Autodesk Inventor part; units mm, degrees
ref_plane "YZ Plane" through (0, 0, 0) normal (1, 0, 0) x (0, 1, 0)
ref_plane "XZ Plane" through (0, 0, 0) normal (0, 1, 0) x (-1, 0, 0)
ref_plane "XY Plane" through (0, 0, 0) normal (0, 0, 1) x (1, 0, 0)
sketch "Sketch1" plane through (0, 0, 0) normal (0, 1, 0) x (-1, 0, 0)
  line L0 (4.0726, -0.3796) -> (56.5523, -0.3796) construction
  line L1 (56.5523, -0.3796) -> (56.5523, -20.3796) construction
  line L2 (56.5523, -20.3796) -> (4.0726, -20.3796) construction
  line L3 (4.0726, -20.3796) -> (4.0726, -0.3796) construction
  line L4 (20.1018, -0.3796) -> (13.3433, -11.5303)
  line L5 (13.3433, -11.5303) -> (13.3433, -20.3796)
  line L6 (13.3433, -20.3796) -> (10.6852, -20.3796)
  line L7 (10.6852, -20.3796) -> (10.6852, -11.8059)
  line L8 (10.6852, -11.8059) -> (3.9267, -0.3796)
  line L9 (3.9267, -0.3796) -> (6.8765, -0.3796)
  line L10 (6.8765, -0.3796) -> (12.0305, -9.1803)
  line L11 (12.0305, -9.1803) -> (17.2817, -0.3796)
  line L12 (17.2817, -0.3796) -> (20.1018, -0.3796)
  line L13 (39.0969, -20.3796) -> (36.4389, -20.3796)
  line L14 (36.4389, -20.3796) -> (36.4389, -3.1511)
  line L15 (36.4389, -3.1511) -> (31.2201, -14.8691)
  line L16 (31.2201, -14.8691) -> (29.5993, -14.8691)
  line L17 (29.5993, -14.8691) -> (24.4292, -3.1511)
  line L18 (24.4292, -3.1511) -> (24.4292, -20.3796)
  line L19 (24.4292, -20.3796) -> (21.9494, -20.3796)
  line L20 (21.9494, -20.3796) -> (21.9494, -0.3796)
  line L21 (21.9494, -0.3796) -> (25.5799, -0.3796)
  line L22 (25.5799, -0.3796) -> (30.5718, -11.5141)
  line L23 (30.5718, -11.5141) -> (35.4016, -0.3796)
  line L24 (35.4016, -0.3796) -> (39.0969, -0.3796)
  line L25 (39.0969, -0.3796) -> (39.0969, -20.3796)
  line L26 (43.1488, -20.3796) -> (43.1488, -0.3796)
  line L27 (43.1488, -0.3796) -> (55.6609, -0.3796)
  line L28 (55.6609, -0.3796) -> (55.6609, -2.7459)
  line L29 (55.6609, -2.7459) -> (45.8068, -2.7459)
  line L30 (45.8068, -2.7459) -> (45.8068, -8.224)
  line L31 (45.8068, -8.224) -> (54.9964, -8.224)
  line L32 (54.9964, -8.224) -> (54.9964, -10.5903)
  line L33 (54.9964, -10.5903) -> (45.8068, -10.5903)
  line L34 (45.8068, -10.5903) -> (45.8068, -18.0133)
  line L35 (45.8068, -18.0133) -> (55.6609, -18.0133)
  line L36 (55.6609, -18.0133) -> (55.6609, -20.3796)
  line L37 (55.6609, -20.3796) -> (43.1488, -20.3796)
  point P0 (0, 0)
extrude "Extrusion1" add sketch "Sketch1" along normal blind 5
sketch "Sketch2" plane through (0, 5, 0) normal (0, 1, 0) x (1, 0, 0)
  line L0 (-17.2817, 0.3796) -> (-12.0305, 9.1803)
  line L1 (-55.6609, 0.3796) -> (-43.1488, 0.3796)
  line L2 (-17.2817, 0.3796) -> (-20.1018, 0.3796)
  line L3 (-55.6609, 2.7459) -> (-55.6609, 0.3796)
  line L4 (-55.6609, 0.3796) -> (-55.6609, 2.7459)
  line L5 (-55.6609, 2.7459) -> (-16.2934, 2.7459)
  line L6 (-16.2934, 2.7459) -> (-17.3426, 0.3796)
  line L7 (-13.3433, 11.5303) -> (-20.1018, 0.3796)
  line L8 (-20.1018, 0.3796) -> (-24.9933, 0.3796)
  line L9 (-21.9494, 0.3796) -> (-25.5799, 0.3796)
  line L10 (-26.1142, 2.7459) -> (-24.9933, 0.3796)
  line L11 (-55.6609, 0.3796) -> (-38.2567, 0.3796)
  line L12 (-39.0969, 0.3796) -> (-35.4016, 0.3796)
  line L13 (-38.2567, 2.7459) -> (-49.9322, 2.7459)
  line L14 (-38.2567, 0.3796) -> (-38.2567, 2.7459)
  point P0 (0, 0)
extrude "Extrusion2" add sketch "Sketch2" against normal blind 5
sketch "Sketch3" plane through (0, 5, 0) normal (0, 1, 0) x (1, 0, 0)
  line L0 (-6.8765, 0.3796) -> (-3.9267, 0.3796)
  line L1 (-6.8765, 0.3796) -> (-1.8765, 0.3796)
  line L2 (-1.8765, 0.3796) -> (-1.8765, 5.3796)
  line L3 (-1.8765, 5.3796) -> (-6.8765, 5.3796)
  line L4 (-6.8765, 5.3796) -> (-6.8765, 0.3796)
  point P0 (0, 0)
  dimension "d9" = 5
  dimension "d10" = 5
extrude "Extrusion3" add sketch "Sketch3" against normal blind 5
sketch "Sketch4" plane through (0, 5, 0) normal (0, 1, 0) x (1, 0, 0)
  circle A0 centre (-4.3765, 2.8796) radius 1.5
  line L0 (-6.8765, 0.3796) -> (-1.8765, 0.3796)
  line L1 (-1.8765, 0.3796) -> (-1.8765, 5.3796)
  point P0 (0, 0)
  dimension "d6" = 2.5
  dimension "d11" = 2.5
  dimension "d12" = 3
extrude "Extrusion4" cut sketch "Sketch4" against normal blind 5
properties part number "YME"
The listing builds one solid part. Answer for the finished solid, in the listing's coordinates (mm). A direction names the side the tool comes from. Give positions to 0.01 mm unless a question says otherwise; leave off trailing zeros. Write each loop counter-clockwise with the first axis right and the second up, starting at its lowest first coordinate (ties: lowest second). Pieces come first, ordered by that corner, then holes. Notation, with made-up numbers: (-1, 85.25) -> (34, 85.25) arc R22 cw to (34, 122.25) -> close; hole circle Ø6 at (14.25, 47). An arc over 180 degrees is marked (long way). Write item = value, one per line. Start each with the question number.
1) The part is cut by section B-B, the plane z = -15.75. Determine the outline of the cut face in (x, y).
2) The part is cut by section D-D, the plane x = -20.5. Determine the outline of the cut face in (y, z), and give its area (3 significant figures).
3) The part is cut by section A-A, the plane x = -52. Determine the outline of the cut face in (y, z).
4) The part is cut by section C-C, the plane z = -13.25. Determine the outline of the cut face in (x, y), and give its area (3 significant figures).
5) Straight lines are drawn through the part: line 1 along Z through (x, y) = (-50, 3.6); line 2 along X through (y, z) = (2.85, -18.75); line 3 along X through (y, z) = (1.7, -17). For each, find the intervals that lie inside material, in ascending order.
6) Each of these flat-tipped pins is pushed along its axis until it touches: pin 1 (2.5 mm diameter, centred on y = 3, z = -9, fed in from -X); pin 2 (1.5 mm diameter, centred on y = 3, z = -14.5, fed in from -X); pin 3 (3 mm diameter, centred on x = -12.5, y = 3.5, fed in from +Z). Where does it stop, or does it pass through?
7) Which of the six approach directions +Z, -Z, +X, -X, +Y, -Y give full straight-line access (tool end or side, diameter ignored) to faces 1 (the face through (-16.04, 2.46, -7.08)), 2 (the face through (-14.62, 2.46, -4.84)), 3 (the face through (-50, 2, -10.59)), 4 (the face through (-12, 2, -20.38))?
Solutions:
q1.outline = (-45.81, 0) -> (-43.15, 0) -> (-43.15, 5) -> (-45.81, 5) -> close; (-39.1, 0) -> (-36.44, 0) -> (-36.44, 5) -> (-39.1, 5) -> close; (-24.43, 0) -> (-21.95, 0) -> (-21.95, 5) -> (-24.43, 5) -> close; (-13.34, 0) -> (-10.69, 0) -> (-10.69, 5) -> (-13.34, 5) -> close
q2.outline = (0, -2.75) -> (5, -2.75) -> (5, -0.38) -> (0, -0.38) -> close
q2.area = 11.8 mm²
q3.outline = (0, -20.38) -> (5, -20.38) -> (5, -18.01) -> (0, -18.01) -> close; (0, -10.59) -> (5, -10.59) -> (5, -8.22) -> (0, -8.22) -> close; (0, -2.75) -> (5, -2.75) -> (5, -0.38) -> (0, -0.38) -> close
q4.outline = (-45.81, 0) -> (-43.15, 0) -> (-43.15, 5) -> (-45.81, 5) -> close; (-39.1, 0) -> (-36.44, 0) -> (-36.44, 5) -> (-39.1, 5) -> close; (-31.94, 0) -> (-28.88, 0) -> (-28.88, 5) -> (-31.94, 5) -> close; (-24.43, 0) -> (-21.95, 0) -> (-21.95, 5) -> (-24.43, 5) -> close; (-13.34, 0) -> (-10.69, 0) -> (-10.69, 5) -> (-13.34, 5) -> close
q4.area = 67.6 mm²
q5.line_1 = -20.38 to -18.01, -10.59 to -8.22, -2.75 to -0.38
q5.line_2 = -55.66 to -43.15, -39.1 to -36.44, -24.43 to -21.95, -13.34 to -10.69
q5.line_3 = -45.81 to -43.15, -39.1 to -36.44, -24.43 to -21.95, -13.34 to -10.69
q6.pin_1 = -55
q6.pin_2 = -45.81
q6.pin_3 = -5.88
q7.face_1 = -Z, +Y, -Y
q7.face_2 = +Z, +Y, -Y
q7.face_3 = -X, +Y, -Y
q7.face_4 = -Z, +X, -X, +Y, -Y
